Verification items for the finished model (mm, model axes). Round coordinates to 2 decimals unless told otherwise and drop trailing zeros. Order: outer loops, then holes, each group sorted by start corner. A loop starts at its lowest first (then second) coordinate and runs counter-clockwise, first axis right, second up. Notation, with made-up numbers: M 69,-12 L 98,-12 A17 cw 98,-8 Z; hole C 17,-39.5 d7. An arc over 180 degrees is marked long. Use CSV: the item, a comma, the result in double quotes. Start each with the question number.
Q1. Gauge pin test, flat ends, axial feed: pin 1 Ø3 at (x, y) = (81.5, 1.5) entering from -Z; pin 2 Ø3 at (x, y) = (111, 2.5) entering from -Z; pin 3 Ø3 at (y, z) = (2.5, -111.5) entering from +X. Record the tip position at first contact, or that the pin passes through.
Q2. Sectioned sample at A-A (y = 1.75). Enter the section's corners in (x, z).
Q3. Scan lines: line 1 (Z direction, x = 106, y = 4.25); line 2 (Z direction, x = 186, y = 4.75); line 3 (X direction, y = 3.75, z = -119.5). Record each from-to range of solid material in increasing order.
```python
from build123d import *

# Parameters (mm, degrees)
BOSS_EXTRUDE1_DEPTH = 7.5
FILLET1_R           = 5
CHAMFER1_SIZE       = 1
SKETCH2_W           = 198
SKETCH2_H           = 149
CUT_EXTRUDE1_DEPTH  = 0.0001


with BuildPart() as part:
    # Sketch1 → Boss-Extrude1 (new body)
    with BuildSketch(Plane(origin=(0, 0, 0), x_dir=(1, 0, 0), z_dir=(0, 1, 0))):
        with BuildLine():
            Line((5, 0), (235, 0))
            ThreePointArc((235, 0), (238.535533906, 1.464466094), (240, 5))
            Line((240, 5), (240, 165))
            ThreePointArc((240, 165), (238.535533906, 168.535533906), (235, 170))
            Line((235, 170), (5, 170))
            ThreePointArc((5, 170), (1.464466094, 168.535533906), (0, 165))
            Line((0, 165), (0, 5))
            ThreePointArc((0, 5), (1.464466094, 1.464466094), (5, 0))
        make_face()
    extrude(amount=BOSS_EXTRUDE1_DEPTH)

    # Fillet1
    fillet1_edges = [part.edges().sort_by_distance(p)[0] for p in [
        (120, 0, 0),
        (1.464466094, 0, -1.464466094),
        (0, 0, -85),
        (1.464466094, 0, -168.535533906),
        (120, 0, -170),
        (238.535533906, 0, -168.535533906),
        (240, 0, -85),
        (238.535533906, 0, -1.464466094),
    ]]
    fillet(fillet1_edges, radius=FILLET1_R)

    # Chamfer1
    chamfer1_edges = [part.edges().sort_by_distance(p)[0] for p in [
        (238.535533906, 7.5, -1.464466094),
        (240, 7.5, -85),
        (238.535533906, 7.5, -168.535533906),
        (120, 7.5, -170),
        (1.464466094, 7.5, -168.535533906),
        (0, 7.5, -85),
        (1.464466094, 7.5, -1.464466094),
        (120, 7.5, 0),
    ]]
    chamfer(chamfer1_edges, length=CHAMFER1_SIZE)

    # Sketch2 → Cut-Extrude1 (cut)
    with BuildSketch(Plane(origin=(0, 7.5, 0), x_dir=(1, 0, 0), z_dir=(0, 1, 0))):
        with Locations((120, 85)):
            Rectangle(SKETCH2_W, SKETCH2_H)
    extrude(amount=-CUT_EXTRUDE1_DEPTH, mode=Mode.SUBTRACT)


solid = part.part
```
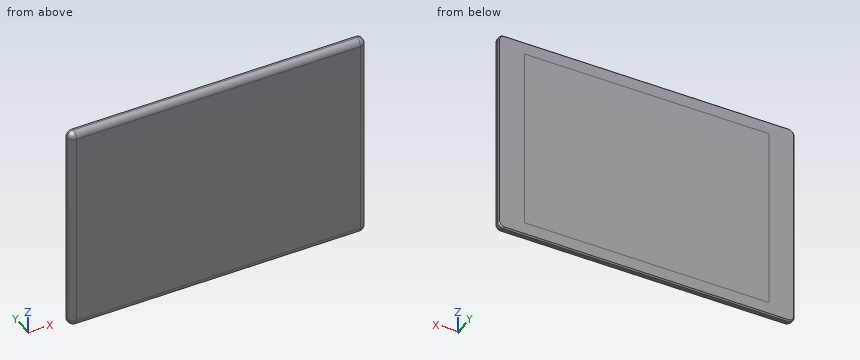
Verdict:
1,pin 1,"stops at z = -169.58"
1,pin 2,"stops at z = -169.9"
1,pin 3,"stops at x = 239.9"
2,outline,"M 1.2,-165 A3.8 ccw 5,-168.8 L 235,-168.8 A3.8 ccw 238.8,-165 L 238.8,-5 A3.8 ccw 235,-1.2 L 5,-1.2 A3.8 ccw 1.2,-5 Z"
3,line 1,"z = -169.94 to -0.06"
3,line 2,"z = -169.99 to -0.01"
3,line 3,"x = 0.16 to 239.84"
